Source: three-view drawing plus pictorial views. Frame: mm from the lowest corner of the part. Round coordinates to 2 decimals unless told otherwise and drop trailing zeros. Loops run counter-clockwise (first coordinate to the right, second up) from the corner with the lowest first, then second, coordinate; pieces in that order, holes last. Notation, with made-up numbers: M -22,32 L -6,32 A23 ccw -6,70 Z; hole C 84,77 d10. An arc over 180 degrees is marked long. Write each question's results on one line, items separated by ' | '.
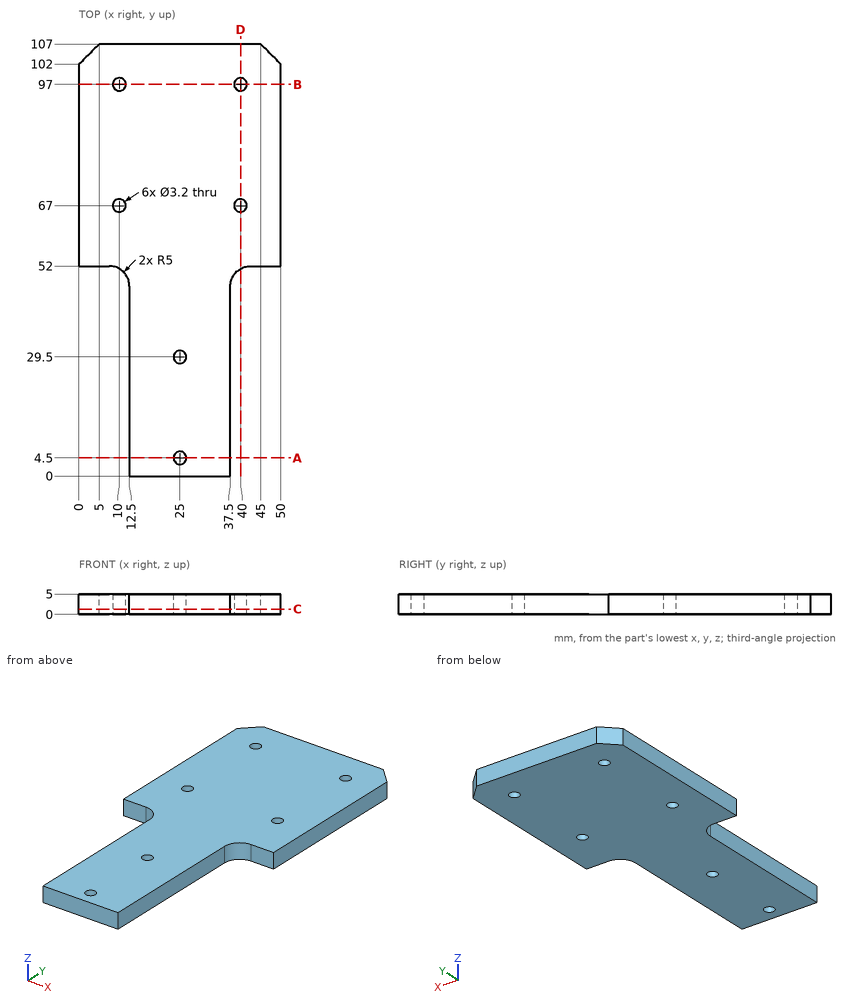
1. Section B-B (y = 97). Output: boundary loops of the cut face in (x, z).
Answer key:
outline: M 0,0 L 8.4,0 L 8.4,5 L 0,5 Z; M 11.6,0 L 38.4,0 L 38.4,5 L 11.6,5 Z; M 41.6,0 L 50,0 L 50,5 L 41.6,5 Z
2. Pin query (flat end, axial travel): P1, Ø1.5, axis at y = 23.5, z = 2.5, coming from the -X side; P2, Ø1.9, axis at x = 10, y = 97, coming from the +Z side. Return the tip coordinate at first contact, or that it passes through.
Answer key:
P1: stops at x = 12.5 | P2: passes through
3. Section A-A (y = 4.5). Output: boundary loops of the cut face in (x, z).
Answer key:
outline: M 12.5,0 L 23.4,0 L 23.4,5 L 12.5,5 Z; M 26.6,0 L 37.5,0 L 37.5,5 L 26.6,5 Z
4. Section C-C (z = 1.25). Output: boundary loops of the cut face in (x, y).
Answer key:
outline: M 0,52 L 7.5,52 A5 cw 12.5,47 L 12.5,0 L 37.5,0 L 37.5,47 A5 cw 42.5,52 L 50,52 L 50,102 L 45,107 L 5,107 L 0,102 Z; hole C 10,67 d3.2; hole C 10,97 d3.2; hole C 25,4.5 d3.2; hole C 25,29.5 d3.2; hole C 40,67 d3.2; hole C 40,97 d3.2
5. Section D-D (x = 40). Output: boundary loops of the cut face in (y, z), then the cut area to 3 significant figures.
Answer key:
outline: M 51.33,0 L 65.4,0 L 65.4,5 L 51.33,5 Z; M 68.6,0 L 95.4,0 L 95.4,5 L 68.6,5 Z; M 98.6,0 L 107,0 L 107,5 L 98.6,5 Z | area: 246 mm²
6. Ray query, probe 1 along X at (y, z) = (67, 3.1); probe 2 along Y at (x, z) = (40, 2.8); probe 3 along Y at (x, z) = (40.5, 1.3). Return the intervals inside material, ascending.
Answer key:
probe 1: x = 0 to 8.4, 11.6 to 38.4, 41.6 to 50 | probe 2: y = 51.33 to 65.4, 68.6 to 95.4, 98.6 to 107 | probe 3: y = 51.58 to 65.48, 68.52 to 95.48, 98.52 to 107
